For this review, take the finished solid that the model builds, in its own axes (mm). A direction names the side the tool comes from. Round coordinates to 2 decimals unless told otherwise and drop trailing zeros. Loops run counter-clockwise (first coordinate to the right, second up) from the corner with the lowest first, then second, coordinate; pieces in that order, holes last. Notation, with made-up numbers: M 41,16.5 L 84,16.5 A18 cw 84,28.5 Z; hole C 50,57.5 d9. An arc over 180 degrees is marked long. One line per question, with ' | ' between items. Start each with the question number.
1) We need section B-B (y = 2.2). State how many separate pieces and enclosed holes the cut face has, and give its area (3 significant figures).
2) We need section D-D (z = -1.75). Give the boundary of the cut face in (x, y), and give its area (3 significant figures).
3) Mouldability with a two-part tool opening along X and no side actions: class faces 6 (the face through (0, 4, 10)), 7 (the face through (3.992, 2.169, -4.227)), 8 (the face through (6.5, 2, 0)) as pulls with the +X half, pulls with the -X half, needs draft (parallel to the pull), parting line crosses it, or undercut.
4) We need section C-C (x = -5.75). Give the boundary of the cut face in (y, z), and give its area (3 significant figures).
5) For pin 1 Ø0.6 at (y, z) = (2.5, -0.5) entering from +X; pin 2 Ø1.2 at (y, z) = (3, -0.5) entering from +X; pin 3 Ø3 at (x, z) = (0, 3) entering from +Y; pin 4 Ø0.7 at (y, z) = (2, 1) entering from -X, all flat-tipped, find the tip position at first contact; note any pin that passes through.
6) For probe 1 along X at (y, z) = (3.8, 5.25); probe 2 along X at (y, z) = (0.8, 5.25); probe 3 along Z at (x, y) = (0.75, 3.7), list the stretches that pass through material, from the lowest coordinate up. Write a range as from..to.
7) We need section A-A (z = 5). Give the boundary of the cut face in (x, y), and give its area (3 significant figures).
8) For faces 1 (the face through (0, 4.4, 0)), 2 (the face through (5.5, 2, 5)), 3 (the face through (6.215, 1.724, -8.699)), 4 (the face through (0, 4, -10)), 5 (the face through (0, 2, -9)), list the 3-axis set-ups (+Z, -Z, +X, -X, +Y, -Y) from which the entire face can be reached by the end or side of a thin tool; tool diameter is ignored.
```python
from build123d import *

# Parameters (mm, degrees)
SKETCH1_W           = 13
SKETCH1_H           = 18
BOSS_EXTRUDE1_DEPTH = 3.4
SKETCH2_W           = 15
SKETCH2_H           = 20
BOSS_EXTRUDE2_DEPTH = 1
SKETCH4_R           = 1.6
CUT_EXTRUDE2_DEPTH  = 14.251792332
FILLET1_R           = 1


with BuildPart() as part:
    # Sketch1 → Boss-Extrude1 (new body)
    with BuildSketch(Plane(origin=(0, 0, 0), x_dir=(1, 0, 0), z_dir=(0, 1, 0))):
        Rectangle(SKETCH1_W, SKETCH1_H)
    extrude(amount=BOSS_EXTRUDE1_DEPTH)

    # Sketch2 → Boss-Extrude2 (add)
    with BuildSketch(Plane(origin=(0, 3.4, 0), x_dir=(1, 0, 0), z_dir=(0, 1, 0))):
        Rectangle(SKETCH2_W, SKETCH2_H)
    extrude(amount=BOSS_EXTRUDE2_DEPTH)

    # Sketch4 → Cut-Extrude2 (cut, through all)
    with BuildSketch(Plane.XZ):
        with BuildLine():
            Line((-2.5, 5.5), (-3.844272635, 6.844272635))
            ThreePointArc((-3.844272635, 6.844272635), (0, 7.85), (3.844272635, 6.844272635))
            Line((3.844272635, 6.844272635), (2.5, 5.5))
            Line((2.5, 5.5), (2.5, 2.5))
            ThreePointArc((2.5, 2.5), (2.758819045, 2.465925826), (3, 2.366025404))
            ThreePointArc((3, 2.366025404), (4, 2.366025404), (4.5, 3.232050808))
            ThreePointArc((4.5, 3.232050808), (4.792893219, 3.939157589), (5.5, 4.232050808))
            Line((5.5, 4.232050808), (5.5, 5.809475019))
            ThreePointArc((5.5, 5.809475019), (0, 8), (-5.5, 5.809475019))
            Line((-5.5, 5.809475019), (-5.5, 3.50401717))
            ThreePointArc((-5.5, 3.50401717), (-4.08113883, 4.211123951), (-2.5, 4.096376317))
            Line((-2.5, 4.096376317), (-2.5, 5.5))
        make_face()
        with BuildLine():
            Line((-2.5, -0.403623683), (-2.5, 2))
            ThreePointArc((-2.5, 2), (-2.758819045, 2.034074174), (-3, 2.133974596))
            ThreePointArc((-3, 2.133974596), (-4, 2.133974596), (-4.5, 1.267949192))
            ThreePointArc((-4.5, 1.267949192), (-4.792893219, 0.560842411), (-5.5, 0.267949192))
            Line((-5.5, 0.267949192), (-5.5, -0.99598283))
            ThreePointArc((-5.5, -0.99598283), (-4.08113883, -0.288876049), (-2.5, -0.403623683))
        make_face()
        with Locations(Location((0, 3, 0), (0, 0, 270))):
            Circle(SKETCH4_R)
        with BuildLine():
            ThreePointArc((5.5, 0.99598283), (4.08113883, 0.288876049), (2.5, 0.403623683))
            Line((2.5, 0.403623683), (2.5, -2))
            ThreePointArc((2.5, -2), (2.758819045, -2.034074174), (3, -2.133974596))
            ThreePointArc((3, -2.133974596), (4, -2.133974596), (4.5, -1.267949192))
            ThreePointArc((4.5, -1.267949192), (4.792893219, -0.560842411), (5.5, -0.267949192))
            Line((5.5, -0.267949192), (5.5, 0.99598283))
        make_face()
        with BuildLine():
            Line((-2.5, -3), (-2.5, -2.5))
            ThreePointArc((-2.5, -2.5), (-2.758819045, -2.465925826), (-3, -2.366025404))
            ThreePointArc((-3, -2.366025404), (-4, -2.366025404), (-4.5, -3.232050808))
            ThreePointArc((-4.5, -3.232050808), (-4.792893219, -3.939157589), (-5.5, -4.232050808))
            Line((-5.5, -4.232050808), (-5.5, -8))
            Line((-5.5, -8), (-0.651664446, -8))
            ThreePointArc((-0.651664446, -8), (-1.569721359, -6.823531152), (-1.994806392, -5.393073127))
            ThreePointArc((-1.994806392, -5.393073127), (-1.967548056, -5.03860077), (-1.817997773, -4.716066461))
            ThreePointArc((-1.817997773, -4.716066461), (-2.323251432, -3.923310773), (-2.5, -3))
        make_face()
        with BuildLine():
            ThreePointArc((5.5, -3.50401717), (3.967891244, -4.231237532), (2.286254496, -4.011454587))
            ThreePointArc((2.286254496, -4.011454587), (1.385482489, -5.080970512), (0.051275139, -5.499474117))
            ThreePointArc((0.051275139, -5.499474117), (0.77025343, -6.581403062), (2, -7))
            ThreePointArc((2, -7), (2.707106781, -7.292893219), (3, -8))
            Line((3, -8), (5.5, -8))
            Line((5.5, -8), (5.5, -3.50401717))
        make_face()
        with Locations(Location((0, -3, 0), (0, 0, 270))):
            Circle(SKETCH4_R)
    extrude(amount=-CUT_EXTRUDE2_DEPTH, mode=Mode.SUBTRACT)

    # Fillet1
    fillet1_edges = [part.edges().sort_by_distance(p)[0] for p in [
        (6.5, 1.7, 9),
        (-6.5, 1.7, 9),
        (-6.5, 1.7, -9),
        (6.5, 1.7, -9),
    ]]
    fillet(fillet1_edges, radius=FILLET1_R)


solid = part.part
```
Answers below:
1) separate pieces: 1 | enclosed holes: 7 | area: 153 mm^2
2) outline: M -7.5,3.4 L -6.5,3.4 L -6.5,0 L -1,0 L -1,4.4 L -7.5,4.4 Z; M 1,0 L 2.5,0 L 2.5,4.4 L 1,4.4 Z; M 4.38,0 L 6.5,0 L 6.5,3.4 L 7.5,3.4 L 7.5,4.4 L 4.38,4.4 Z | area: 42.2 mm^2
3) face 6: needs draft | face 7: undercut | face 8: pulls with the +X half
4) outline: M 0,-8.97 L 3.4,-8.97 L 3.4,-10 L 4.4,-10 L 4.4,10 L 3.4,10 L 3.4,8.97 L 0,8.97 Z | area: 81.0 mm^2
5) pin 1: x = 6.5 | pin 2: x = 7.5 | pin 3: through | pin 4: x = -6.5
6) probe 1: -7.5..-5.5, -2.5..2.5, 5.5..7.5 | probe 2: -6.5..-5.5, -2.5..2.5, 5.5..6.5 | probe 3: -10..-6.57, -5.38..-4.41, -1.59..1.59, 4.41..7.81, 7.96..10
7) outline: M -7.5,3.4 L -6.5,3.4 L -6.5,0 L -5.5,0 L -5.5,4.4 L -7.5,4.4 Z; M -2.5,0 L 2.5,0 L 2.5,4.4 L -2.5,4.4 Z; M 5.5,0 L 6.5,0 L 6.5,3.4 L 7.5,3.4 L 7.5,4.4 L 5.5,4.4 Z | area: 32.8 mm^2
8) face 1: +Z, -Z, +X, -X, +Y | face 2: +Y, -Y | face 3: -Z, +X, -Y | face 4: -Z, +X, -X, +Y, -Y | face 5: -Z, +X, -X, -Y
